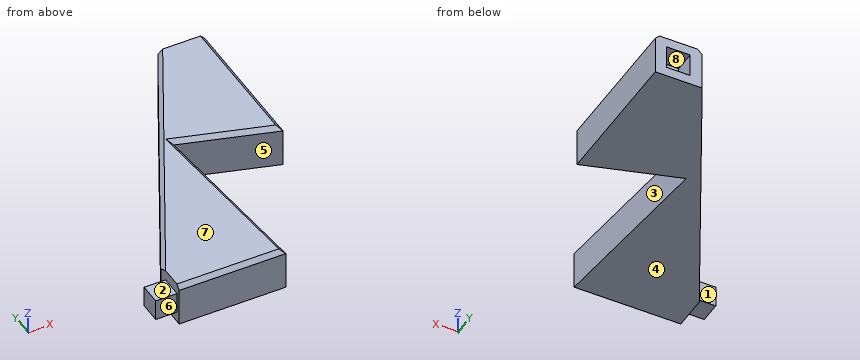
from build123d import *

# Parameters (mm, degrees)
F1_DEPTH = 10
F2_SIZE  = 1
F3_W     = 2.5
F3_H     = 5
F4_DEPTH = 5
F5_W     = 2.75
F5_H     = 5.5
F6_DEPTH = 5


with BuildPart() as f1:
    # F0 (on Top) → F1 (new body)
    with BuildSketch(Plane.XY):
        Polygon((32.334468, 61.115628), (0, 0), (0, -8), (25, -8), (21.339459, 33.840177), (43.334468, 27.115628), (43.334468, 61.115628), align=None)
    extrude(amount=F1_DEPTH)

    # F2
    f2_edges = [f1.edges().sort_by_distance(p)[0] for p in [
        (16.167234, 30.557814, 10),
        (12.5, -8, 10),
        (23.169729, 12.920089, 10),
        (32.336963, 30.477903, 10),
        (43.334468, 44.115628, 10),
    ]]
    chamfer(f2_edges, length=F2_SIZE)

    # F3 (on face) → F4 (join)
    with BuildSketch(Plane(origin=(0, 0, 0), x_dir=(0, -1, 0), z_dir=(-1, 0, 0))):
        with Locations((5.819171, 5)):
            Rectangle(F3_W, F3_H)
        with Locations((3.319171, 5)):
            Rectangle(F3_W, F3_H)
    extrude(amount=F4_DEPTH)

    # F5 (on face) → F6 (cut)
    with BuildSketch(Plane(origin=(0, 61.115628, 0), x_dir=(-1, 0, 0), z_dir=(0, 1, 0))):
        with Locations((-36.525135, 5)):
            Rectangle(F5_W, F5_H)
        with Locations((-39.275135, 5)):
            Rectangle(F5_W, F5_H)
    extrude(amount=-F6_DEPTH, mode=Mode.SUBTRACT)


solid = f1.part
Could you check a few things on this model? Use its own coordinates, in mm. Face numbers are marked on the shaded views. A direction names the side the tool comes from. Coordinates: 2 decimals unless noted, no trailing zeros. Order: outer loops, then holes, each group sorted by start corner. A loop starts at its lowest first (then second) coordinate and runs counter-clockwise, first axis right, second up. Notation, with made-up numbers: (81, -10) -> (116, -10) arc R16 cw to (116, 17) -> close; hole circle Ø7 at (84.25, 39). An arc over 180 degrees is marked (long way). One line per item, written item: value. Start each with the question number.
1) Imagine slicing it at A-A on z = 4. List the corners of the cut face in (x, y) for me, plus the area to 3 significant figures.
2) We'd pull the mould along Y, two halves only. Please class the marked faces 1, 2 and 3: +Y half, -Y half, draft (parallel to the pull), parting line (faces both ways), or undercut.
3) Imagine slicing it at D-D on y = 48. List the corners of the cut face in (x, z) for me, plus the area to 3 significant figures.
4) Which directions (+Z, -Z, +X, -X, +Y, -Y) give clear straight access to the entire face, cutting with the end or side of a thin tool? Please do the marked faces 4, 5, 6, 7 and 8.
5) If I drill on L1, parallel to X at y = 57.5, z = 6.25; L2, parallel to Y at x = 6.5, z = 5.5; L3, parallel to X at y = 9.5, z = 6.75, over which ranges is the centre line in solid material (lowest first)? Write a range as [from, to].
6) I'm going to push flat-ended pins straight in: pin 1 (4 mm diameter, centred on x = 3, z = 5, fed in from +Y); pin 2 (1 mm diameter, centred on y = 27.5, z = 4.5, fed in from -X); pin 3 (2.5 mm diameter, centred on x = -3, y = -4, fed in from -Z). Where does each tip first touch, or does it pass through?
7) Imagine slicing it at B-B on y = 33. List the corners of the cut face in (x, z) for me, plus the area to 3 significant figures.
8) Imagine slicing it at C-C on x = 16.5. List the corners of the cut face in (y, z) for me, plus the area to 3 significant figures.
Answer list:
1. outline: (-5, -7.07) -> (0, -7.07) -> (0, -8) -> (25, -8) -> (21.34, 33.84) -> (43.33, 27.12) -> (43.33, 61.12) -> (40.65, 61.12) -> (40.65, 56.12) -> (35.15, 56.12) -> (35.15, 61.12) -> (32.33, 61.12) -> (0, 0) -> (0, -2.07) -> (-5, -2.07) -> close
1. area: 1,230 mm2
2. face 1: +Y half
2. face 2: draft
2. face 3: undercut
3. outline: (25.4, 0) -> (43.33, 0) -> (43.33, 9) -> (42.33, 10) -> (26.53, 10) -> (25.4, 9) -> close
3. area: 178 mm2
4. face 4: -Z, +X, -X, +Y, -Y
4. face 5: +Z, -Z
4. face 6: +Z, -Z, -X, -Y
4. face 7: +Z, +X, -X, +Y, -Y
4. face 8: +Y
5. L1: x = [30.42, 35.15], [40.65, 43.33]
5. L2: y = [-8, 12.29]
5. L3: x = [5.03, 23.47]
6. pin 1: stops at y = 9.45
6. pin 2: stops at x = 14.28
6. pin 3: stops at z = 2.5
7. outline: (17.46, 0) -> (21.41, 0) -> (21.41, 9) -> (20.41, 10) -> (18.59, 10) -> (17.46, 9) -> close; (24.09, 0) -> (43.33, 0) -> (43.33, 9) -> (42.33, 10) -> (27.51, 10) -> (24.09, 9) -> close
7. area: 229 mm2
8. outline: (-8, 0) -> (31.19, 0) -> (31.19, 9) -> (29.05, 10) -> (-7, 10) -> (-8, 9) -> close
8. area: 390 mm2
